Geometry check sheet. Reference: the model listing, model coordinates, mm. Face numbers are marked on the shaded views. A direction names the side the tool comes from. Give positions to 0.01 mm unless a question says otherwise; leave off trailing zeros. Loops run counter-clockwise (first coordinate to the right, second up) from the corner with the lowest first, then second, coordinate; pieces in that order, holes last. Notation, with made-up numbers: (-14, -24) -> (6, -24) arc R27 cw to (6, 2) -> close; hole circle Ø1 at (71, -34). An arc over 180 degrees is marked (long way). Write item = value, one per line.
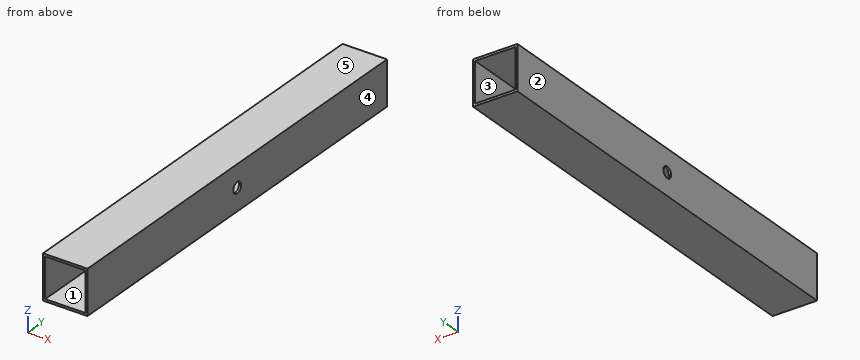
```python
from build123d import *

# Parameters (mm, degrees)
SKETCH1_W               = 20
SKETCH1_H               = 20
SKETCH1_W_2             = 18
SKETCH1_H_2             = 18
BOSS_EXTRUDE1_DEPTH     = 191
CUT_EXTRUDE1_DEPTH      = 193.304446126
CUT_EXTRUDE1_DEPTH_BACK = 193.304446126
SKETCH2_R               = 2.5


with BuildPart() as part:
    # Sketch1 → Boss-Extrude1 (new body)
    with BuildSketch(Plane(origin=(0, 0, 0), x_dir=(1, 0, 0), z_dir=(0, 1, 0))):
        Rectangle(SKETCH1_W, SKETCH1_H)
        Rectangle(SKETCH1_W_2, SKETCH1_H_2, mode=Mode.SUBTRACT)
    extrude(amount=BOSS_EXTRUDE1_DEPTH)

    # Sketch2 → Cut-Extrude1 (cut, two sides: drawn at the far end of the back side and taken through both)
    with BuildSketch(Plane.ZY.offset(10).offset(-CUT_EXTRUDE1_DEPTH_BACK)):
        with Locations(Location((0, 95.5, 0), (0, 0, 180))):
            Circle(SKETCH2_R)
    extrude(amount=CUT_EXTRUDE1_DEPTH + CUT_EXTRUDE1_DEPTH_BACK, mode=Mode.SUBTRACT)


solid = part.part
```
Item 1: Tool access check on the marked faces 1 and 2. Record the directions out of +Z, -Z, +X, -X, +Y, -Y that give a thin tool (end or side, any length) a straight path to the whole face; none if there is none.
Answer:
face_1 = +Y, -Y
face_2 = +Z, -Z, -X, +Y, -Y
Item 2: Section check C-C, the plane x = 0.25. Record the cut outline in (y, z).
Answer:
outline = (0, -10) -> (191, -10) -> (191, -9) -> (0, -9) -> close; (0, 9) -> (191, 9) -> (191, 10) -> (0, 10) -> close
Item 3: Draft check along Z on the marked faces 3, 4 and 5. Enter one of: +Z half, -Z half, draft (parallel to the pull), parting line (faces both ways), or undercut.
Answer:
face_3 = undercut
face_4 = draft
face_5 = +Z half
Item 4: Section check A-A, the plane z = 0. Record the cut outline in (x, y).
Answer:
outline = (-10, 0) -> (-9, 0) -> (-9, 93) -> (-10, 93) -> close; (-10, 98) -> (-9, 98) -> (-9, 191) -> (-10, 191) -> close; (9, 0) -> (10, 0) -> (10, 93) -> (9, 93) -> close; (9, 98) -> (10, 98) -> (10, 191) -> (9, 191) -> close
Item 5: Section check B-B, the plane y = 112. Record the cut outline in (x, z), plus the area to 3 significant figures.
Answer:
outline = (-10, -10) -> (10, -10) -> (10, 10) -> (-10, 10) -> close; hole (-9, -9) -> (9, -9) -> (9, 9) -> (-9, 9) -> close
area = 76.0 mm^2
Item 6: Thickness scan on L1, parallel to X at y = 177.5, z = 4.75; L2, parallel to Y at x = -9.3, z = 0. Record the ranges inside material, lowest first. Write a range as [from, to].
Answer:
L1 = [-10, -9], [9, 10]
L2 = [0, 93], [98, 191]
